```python
from build123d import *

# Parameters (mm, degrees)
SKETCH1_W           = 59.69
SKETCH1_H           = 0.5
EXTRUDE_THIN1_DEPTH = 10
SKETCH3_OUTSIDE_W   = 73.794
SKETCH3_OUTSIDE_H   = 24.104
SKETCH3_OUTSIDE_W_2 = 59.69
SKETCH3_OUTSIDE_H_2 = 10
CUT_EXTRUDE5_DEPTH  = 2.54


with BuildPart() as part:
    # Sketch1 → Extrude-Thin1 (new body)
    with BuildSketch(Plane.XY):
        with Locations((29.845, -0.25)):
            Rectangle(SKETCH1_W, SKETCH1_H)
    extrude(amount=EXTRUDE_THIN1_DEPTH)

    # Sketch3 outside → Cut-Extrude5 (cut)
    # profile 1 of 3: a face of its own
    with BuildSketch(Plane(origin=(0, 0, 0), x_dir=(1, 0, 0), z_dir=(0, 1, 0))):
        with Locations((29.845, -5)):
            Rectangle(SKETCH3_OUTSIDE_W, SKETCH3_OUTSIDE_H)
        with Locations((29.845, -5)):
            Rectangle(SKETCH3_OUTSIDE_W_2, SKETCH3_OUTSIDE_H_2, mode=Mode.SUBTRACT)
    # profile 2 of 3: a face of its own
    with BuildSketch(Plane(origin=(0, 0, 0), x_dir=(1, 0, 0), z_dir=(0, 1, 0))):
        with BuildLine():
            Line((32.004, -2.968), (38.608, -2.968))
            ThreePointArc((38.608, -2.968), (40.64, -5), (38.608, -7.032))
            Line((38.608, -7.032), (32.004, -7.032))
            ThreePointArc((32.004, -7.032), (29.972, -5), (32.004, -2.968))
        make_face()
    # profile 3 of 3: a face of its own
    with BuildSketch(Plane(origin=(0, 0, 0), x_dir=(1, 0, 0), z_dir=(0, 1, 0))):
        with BuildLine():
            Line((49.911, -2.968), (56.515, -2.968))
            ThreePointArc((56.515, -2.968), (58.547, -5), (56.515, -7.032))
            Line((56.515, -7.032), (49.911, -7.032))
            ThreePointArc((49.911, -7.032), (47.879, -5), (49.911, -2.968))
        make_face()
    extrude(amount=-CUT_EXTRUDE5_DEPTH, mode=Mode.SUBTRACT)


solid = part.part
```
The listing builds one solid part. Answer for the finished solid, in the listing's coordinates (mm). A direction names the side the tool comes from. Coordinates: 2 decimals unless noted, no trailing zeros. Write each loop counter-clockwise with the first axis right and the second up, starting at its lowest first coordinate (ties: lowest second). Pieces come first, ordered by that corner, then holes. Notation, with made-up numbers: (-18, 15) - (24, 15) arc R30 ccw to (24, 38) - close; hole circle Ø9 at (-21, 4). An arc over 180 degrees is marked (long way). One line per item, written item: value.
1) This flat-tipped pin is pushed along its axis until it touches: pin 1 Ø2 at (x, z) = (27.5, 2.5) entering from +Y. Where does it stop, or does it pass through?
Geometry check:
pin 1: stops at y = 0
2) Consider line 1 along X through (y, z) = (-0.4, 3.25); line 2 along X through (y, z) = (-0.1, 5.25); line 3 along Z through (x, y) = (53.5, -0.45). Determine where each line is inside the solid, lowest interval first. Write a range as from..to.
Geometry check:
line 1: x = 0..30.97, 39.64..48.88, 57.55..59.69
line 2: x = 0..29.99, 40.62..47.89, 58.53..59.69
line 3: z = 0..2.97, 7.03..10
3) Find section B-B (y = -0.2). Give the vertices of the cut face in (x, z) (3 decimals), and give its area (3 significant figures).
Geometry check:
outline: (0, 0) - (59.69, 0) - (59.69, 10) - (0, 10) - close; hole (32.004, 2.968) - (38.608, 2.968) arc R2.032 ccw to (38.608, 7.032) - (32.004, 7.032) arc R2.032 ccw to start; hole (49.911, 2.968) - (56.515, 2.968) arc R2.032 ccw to (56.515, 7.032) - (49.911, 7.032) arc R2.032 ccw to start
area: 517 mm2
4) Find section A-A (z = 5). Give the vertices of the cut face in (x, y), and give its area (3 significant figures).
Geometry check:
outline: (0, -0.5) - (29.97, -0.5) - (29.97, 0) - (0, 0) - close; (40.64, -0.5) - (47.88, -0.5) - (47.88, 0) - (40.64, 0) - close; (58.55, -0.5) - (59.69, -0.5) - (59.69, 0) - (58.55, 0) - close
area: 19.2 mm2
5) For a pull along Z with two mould halves and no side action, classify faces 1 (the cylindrical face through (58.547, -0.246, 4.955)), 2 (the flat face through (29, -0.5, 5)) as pulls with the +Z half, pulls with the -Z half, needs draft (parallel to the pull), parting line crosses it, or undercut.
Geometry check:
face 1: undercut
face 2: needs draft
6) A tool of negligible diameter and unlimited length cuts with its end or side. For faces 3 (the flat face through (29, 0, 5)), 4 (the cylindrical face through (40.64, -0.25, 4.96)), from which of +Z, -Z, +X, -X, +Y, -Y can it reach the whole face along a straight path? Write none if from no direction.
Geometry check:
face 3: +Z, -Z, +X, -X, +Y
face 4: +Y, -Y
